Input: part model. Units: mm. Frame: model coordinates. Face numbers are marked on the shaded views. Round coordinates to 2 decimals unless told otherwise and drop trailing zeros. Write each loop counter-clockwise with the first axis right and the second up, starting at its lowest first coordinate (ties: lowest second). Pieces come first, ordered by that corner, then holes. Notation, with made-up numbers: (-3, 71) - (11, 71) arc R17 cw to (11, 78) - close; hole circle Ø10 at (-8.5, 14). An arc over 180 degrees is marked (long way). Use one line per item in the form item = value.
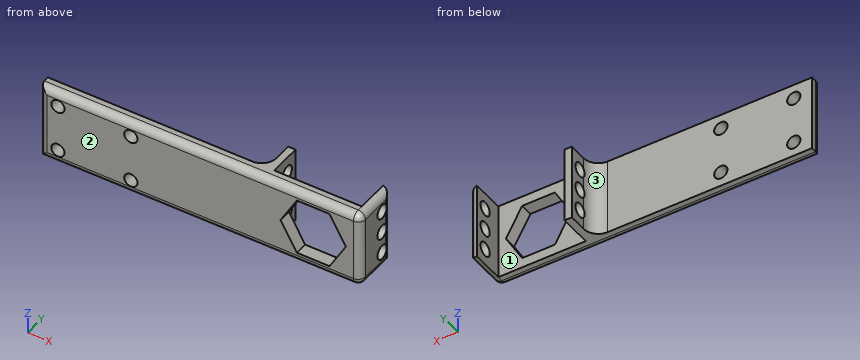
```python
from build123d import *

# Parameters (mm, degrees)
BOSS_EXTRUDE1_DEPTH              = 21
FILLET1_R                        = 4
M3_5_CLEARANCE_HOLE1_D           = 3.9
M3_5_CLEARANCE_HOLE1_CSINK_D     = 3.95
M3_5_CLEARANCE_HOLE1_CSINK_ANGLE = 90
SKETCH4_R                        = 1.825
CUT_EXTRUDE1_DEPTH               = 21
FILLET3_R                        = 2


with BuildPart() as part:
    # Sketch1 → Boss-Extrude1 (new body)
    with BuildSketch(Plane.XY):
        Polygon((12, -20.545429918), (14, -20.545429918), (14, -33.045429918), (-74, -33.045429918), (-74, -29.545429918), (-14, -29.545429918), (-14, -20.545429918), (-12, -20.545429918), (-12, -29.545429918), (12, -29.545429918), align=None)
    extrude(amount=-BOSS_EXTRUDE1_DEPTH)

    # Fillet1
    fillet1_edges = [part.edges().sort_by_distance(p)[0] for p in [
        (-14, -29.545429918, -10.5),
    ]]
    fillet(fillet1_edges, radius=FILLET1_R)

    # M3.5 Clearance Hole1 (through all)
    with Locations(Plane(origin=(14, 0, 0), x_dir=(0, 0, -1), z_dir=(1, 0, 0))):
        with Locations((4.5, -24), (10.5, -24), (16.5, -24)):
            CounterSinkHole(M3_5_CLEARANCE_HOLE1_D / 2, M3_5_CLEARANCE_HOLE1_CSINK_D / 2, counter_sink_angle=M3_5_CLEARANCE_HOLE1_CSINK_ANGLE)

    # Sketch4 → Cut-Extrude1 (cut)
    with BuildSketch(Plane.XZ.offset(33.045429918)):
        with Locations((-69, -4)):
            Circle(SKETCH4_R)
        with Locations((-49, -4)):
            Circle(SKETCH4_R)
        with Locations((18.166214484, -42.778432013)):
            Circle(SKETCH4_R)
        with Locations((28.166214484, -60.098940088)):
            Circle(SKETCH4_R)
        with Locations(Location((-69, -17, 0), (0, 0, 180))):
            Circle(SKETCH4_R)
        with Locations(Location((-49, -17, 0), (0, 0, 180))):
            Circle(SKETCH4_R)
        Polygon((-3.49922334, -18.252792933), (5.452930834, -18.252792933), (9.929007921, -10.5), (5.452930834, -2.747207067), (-3.49922334, -2.747207067), (-7.975300427, -10.5), align=None)
    extrude(amount=-CUT_EXTRUDE1_DEPTH, mode=Mode.SUBTRACT)

    # Fillet3
    # the kernel refuses this fillet: 2 mm, written as the material it takes off along each edge
    with BuildSketch(Plane(origin=(12, -31.045429918, -19), x_dir=(0, 0, -1), z_dir=(0, -1, 0))) as fillet3_piece_1_section:
        Polygon((0, 0), (FILLET3_R, 0), (FILLET3_R, FILLET3_R), (0, FILLET3_R), align=None)
    fillet3_piece_1 = extrude(amount=FILLET3_R, mode=Mode.PRIVATE)
    fillet3_piece_1 = fillet3_piece_1 - Plane(origin=(12, -31.045429918, -19), x_dir=(-0.7071067811865475, 0, 0.7071067811865475), z_dir=(0, -1, 0)) * Sphere(FILLET3_R, mode=Mode.PRIVATE)
    add(fillet3_piece_1, mode=Mode.SUBTRACT)
    with BuildSketch(Plane(origin=(12, -31.045429918, -2), x_dir=(0, -1, 0), z_dir=(0, 0, 1))) as fillet3_piece_2_section:
        Polygon((0, 0), (FILLET3_R, 0), (FILLET3_R, FILLET3_R), (0, FILLET3_R), align=None)
    fillet3_piece_2 = extrude(amount=FILLET3_R, mode=Mode.PRIVATE)
    fillet3_piece_2 = fillet3_piece_2 - Plane(origin=(12, -31.045429918, -2), x_dir=(-0.7071067811865476, 0.7071067811865475, 0), z_dir=(0, 0, 1)) * Sphere(FILLET3_R, mode=Mode.PRIVATE)
    add(fillet3_piece_2, mode=Mode.SUBTRACT)
    with BuildSketch(Plane(origin=(-74, -33.045429918, 5), x_dir=(0, 1, 0), z_dir=(0, 0, -1)), Plane(origin=(14, -20.545429918, 5), x_dir=(0, -1, 0), z_dir=(0, 0, -1))) as fillet3_piece_3:
        with BuildLine():
            CenterArc((FILLET3_R, FILLET3_R), FILLET3_R, 180, 90)
            Line((0, FILLET3_R), (0, 0))
            Line((0, 0), (FILLET3_R, 0))
        make_face()
    extrude(amount=31, mode=Mode.SUBTRACT)
    with BuildSketch(Plane(origin=(12, -33.045429918, -21), x_dir=(0, 1, 0), z_dir=(-1, 0, 0))) as fillet3_piece_4:
        with BuildLine():
            CenterArc((FILLET3_R, -FILLET3_R), FILLET3_R, 90, 90)
            Line((0, -FILLET3_R), (0, 0))
            Line((0, 0), (FILLET3_R, 0))
        make_face()
    extrude(amount=91, mode=Mode.SUBTRACT)
    with BuildSketch(Plane(origin=(12, -33.045429918, 0), x_dir=(0, 1, 0), z_dir=(-1, 0, 0))) as fillet3_piece_5:
        with BuildLine():
            CenterArc((FILLET3_R, FILLET3_R), FILLET3_R, 180, 90)
            Line((0, FILLET3_R), (0, 0))
            Line((0, 0), (FILLET3_R, 0))
        make_face()
    extrude(amount=91, mode=Mode.SUBTRACT)
    with BuildSketch(Plane(origin=(14, -15.545429918, -21), x_dir=(-1, 0, 0), z_dir=(0, -1, 0))) as fillet3_piece_6:
        with BuildLine():
            CenterArc((FILLET3_R, -FILLET3_R), FILLET3_R, 90, 90)
            Line((0, -FILLET3_R), (0, 0))
            Line((0, 0), (FILLET3_R, 0))
        make_face()
    extrude(amount=15.5, mode=Mode.SUBTRACT)
    with BuildSketch(Plane(origin=(14, -15.545429918, 0), x_dir=(-1, 0, 0), z_dir=(0, -1, 0))) as fillet3_piece_7:
        with BuildLine():
            CenterArc((FILLET3_R, FILLET3_R), FILLET3_R, 180, 90)
            Line((0, FILLET3_R), (0, 0))
            Line((0, 0), (FILLET3_R, 0))
        make_face()
    extrude(amount=15.5, mode=Mode.SUBTRACT)
    with BuildSketch(Plane(origin=(14, -33.045429918, -2), x_dir=(-1, 0, 0), z_dir=(0, 0, -1))) as fillet3_piece_8:
        with BuildLine():
            CenterArc((FILLET3_R, FILLET3_R), FILLET3_R, 180, 90)
            Line((0, FILLET3_R), (0, 0))
            Line((0, 0), (FILLET3_R, 0))
        make_face()
    extrude(amount=17, mode=Mode.SUBTRACT)


solid = part.part
```
(1) Cut plane A-A on x = -49. Output: boundary loops of the cut face in (y, z) (3 decimals).
Derived:
outline = (-33.045, -19) arc R2 ccw to (-31.045, -21) - (-29.545, -21) - (-29.545, -18.825) - (-33.045, -18.825) - close; (-33.045, -15.175) - (-29.545, -15.175) - (-29.545, -5.825) - (-33.045, -5.825) - close; (-33.045, -2.175) - (-29.545, -2.175) - (-29.545, 0) - (-31.045, 0) arc R2 ccw to (-33.045, -2) - close
(2) First-contact query: pin 1 Ø4 at (x, z) = (-69, -4) entering from +Y; pin 2 Ø1.5 at (y, z) = (-23, -13.5) entering from -X; pin 3 Ø4.5 at (y, z) = (-24, -10.5) entering from -X. Flat tips, straight axial feed; report the tip coordinate or a pass-through.
Derived:
pin_1 = -29.55
pin_2 = -14
pin_3 = -14.06
(3) Material intervals for L1, parallel to Z at x = -13.45, y = -24; L2, parallel to X at y = -25.5, z = -2.25; L3, parallel to X at y = -27.5, z = -15.25, sorted ascending.
Derived:
L1 = -21 to -18.45, -14.55 to -12.45, -8.55 to -6.45, -2.55 to 0
L2 = -14 to -12, 12 to 14
L3 = -14.51 to -12, 12 to 14
(4) Cut plane C-C on x = -22. Output: boundary loops of the cut face in (y, z).
Derived:
outline = (-33.05, -19) arc R2 ccw to (-31.05, -21) - (-29.55, -21) - (-29.55, 0) - (-31.05, 0) arc R2 ccw to (-33.05, -2) - close
(5) Draft query along X for the marked faces 1, 2 and 3. Return one class per face: released by +X, released by -X, zero draft, split by the parting line, or undercut.
Derived:
face_1 = undercut
face_2 = zero draft
face_3 = released by -X
(6) Cut plane B-B on y = -28.25. Output: boundary loops of the cut face in (x, z).
Derived:
outline = (-15.05, -21) - (-12, -21) - (-12, 0) - (-15.05, 0) - close; (12, -21) arc R2 ccw to (14, -19) - (14, -2) arc R2 ccw to (12, 0) - close
